```python
from build123d import *

# Parameters (mm, degrees)
SKETCH1_R           = 102.87
SKETCH1_R_2         = 6.35
BOSS_EXTRUDE1_DEPTH = 6.35
SKETCH6_R           = 25.4
CUT_EXTRUDE1_DEPTH  = 28.448


with BuildPart() as part:
    # Sketch1 → Boss-Extrude1 (new body)
    with BuildSketch(Plane(origin=(0, 0, 0), x_dir=(1, 0, 0), z_dir=(0, 1, 0))):
        with BuildLine():
            Line((256.521079071, 133.368920929), (0, 133.368920929))
            ThreePointArc((0, 133.368920929), (-94.306068389, 94.306068389), (-133.368920929, 0))
            Line((-133.368920929, 0), (-133.368920929, -95.231079071))
            ThreePointArc((-133.368920929, -95.231079071), (-129.64917705, -104.211335192), (-120.668920929, -107.931079071))
            Line((-120.668920929, -107.931079071), (227.955539535, -107.931079071))
            ThreePointArc((227.955539535, -107.931079071), (230.193914007, -107.003914007), (231.121079071, -104.765539535))
            Line((231.121079071, -104.765539535), (231.121079071, 3.100777109))
            ThreePointArc((231.121079071, 3.100777109), (232.98095101, 7.59090517), (237.471079071, 9.450777109))
            Line((237.471079071, 9.450777109), (256.521079071, 9.450777109))
            ThreePointArc((256.521079071, 9.450777109), (261.011207131, 11.310649048), (262.871079071, 15.800777109))
            Line((262.871079071, 15.800777109), (262.871079071, 127.018920929))
            ThreePointArc((262.871079071, 127.018920929), (261.011207131, 131.50904899), (256.521079071, 133.368920929))
        make_face()
        Circle(SKETCH1_R, mode=Mode.SUBTRACT)
        with Locations((-112.738641363, -14.374963544)):
            Circle(SKETCH1_R_2, mode=Mode.SUBTRACT)
        with Locations((43.920237074, 104.822009181)):
            Circle(SKETCH1_R_2, mode=Mode.SUBTRACT)
        with Locations((68.818404289, -90.447045637)):
            Circle(SKETCH1_R_2, mode=Mode.SUBTRACT)
        with Locations((250.171079071, 107.968920929)):
            Circle(SKETCH1_R_2, mode=Mode.SUBTRACT)
        with Locations((250.171079071, 34.850777109)):
            Circle(SKETCH1_R_2, mode=Mode.SUBTRACT)
    extrude(amount=BOSS_EXTRUDE1_DEPTH)

    # Sketch6 → Cut-Extrude1 (cut)
    with BuildSketch(Plane(origin=(0, 0, 0), x_dir=(1, 0, 0), z_dir=(0, 1, 0))):
        with Locations((173.810939206, 0)):
            Circle(SKETCH6_R)
    extrude(amount=CUT_EXTRUDE1_DEPTH, mode=Mode.SUBTRACT)


solid = part.part
```
Geometry: final body of the model. Coordinates: model frame, mm. Coordinates: 2 decimals unless noted, no trailing zeros. Order: outer loops, then holes, each group sorted by start corner. A loop starts at its lowest first (then second) coordinate and runs counter-clockwise, first axis right, second up. Notation, with made-up numbers: (-22.75, -21) - (12.25, -21) arc R34 ccw to (12.25, 16) - close; hole circle Ø6 at (56, -27). An arc over 180 degrees is marked (long way). Return JSON: item names as keys, results as strings. Group by question number.
1. Pull-direction query (X, two-part tool) for faces 1 (the face through (-129.75, 3.13, 104.11)), 2 (the face through (-109.325, 3.131, 9.021)), 3 (the face through (106, 6.35, -14)); classes: pulls with the +X half, pulls with the -X half, needs draft (parallel to the pull), parting line crosses it, or undercut.
2. Cut plane B-B (y = 2). Output: boundary loops of the cut face in (x, z).
3. Cut plane A-A (z = 47). Output: boundary loops of the cut face in (x, y), plus the area to 3 significant figures.
4. Material intervals for line 1 along X through (y, z) = (2.5, 0); line 2 along Z through (x, y) = (41.5, 2.75); line 3 along X through (y, z) = (4, 2), sorted ascending. Write a range as [from, to].
5. Cut plane C-C (x = -25). Output: boundary loops of the cut face in (y, z).
6. Pin query (flat end, axial travel): pin 1 (3 mm diameter, centred on y = 5.5, z = -11, fed in from -X). Return the tip coordinate at first contact, or that it passes through.
Resolved:
{
 "1": {"face 1": "pulls with the -X half", "face 2": "undercut", "face 3": "needs draft"},
 "2": {"outline": "(-133.37, 0) arc R133.37 ccw to (0, -133.37) - (256.52, -133.37) arc R6.35 ccw to (262.87, -127.02) - (262.87, -15.8) arc R6.35 ccw to (256.52, -9.45) - (237.47, -9.45) arc R6.35 cw to (231.12, -3.1) - (231.12, 104.77) arc R3.17 ccw to (227.96, 107.93) - (-120.67, 107.93) arc R12.7 ccw to (-133.37, 95.23) - close; hole circle Ø12.7 at (-112.74, 14.37); hole circle Ø205.74 at (0, 0); hole circle Ø12.7 at (43.92, -104.82); hole circle Ø12.7 at (68.82, 90.45); hole circle Ø50.8 at (173.81, 0); hole circle Ø12.7 at (250.17, -107.97); hole circle Ø12.7 at (250.17, -34.85)"},
 "3": {"outline": "(-133.37, 0) - (-91.51, 0) - (-91.51, 6.35) - (-133.37, 6.35) - close; (91.51, 0) - (231.12, 0) - (231.12, 6.35) - (91.51, 6.35) - close", "area": "1,150 mm²"},
 "4": {"line 1": "x = [-133.37, -102.87], [102.87, 148.41], [199.21, 231.12]", "line 2": "z = [-133.37, -110.69], [-98.95, -94.13], [94.13, 107.93]", "line 3": "x = [-133.37, -102.85], [102.85, 148.49], [199.13, 231.12]"},
 "5": {"outline": "(0, -131) - (6.35, -131) - (6.35, -99.79) - (0, -99.79) - close; (0, 99.79) - (6.35, 99.79) - (6.35, 107.93) - (0, 107.93) - close"},
 "6": {"pin 1": "stops at x = -133.03"}
}
